The model under review builds one solid part; all positions refer to its coordinate system, in mm. A direction names the side the tool comes from. Coordinates: 2 decimals unless noted, no trailing zeros. Loops run counter-clockwise (first coordinate to the right, second up) from the corner with the lowest first, then second, coordinate; pieces in that order, holes last. Notation, with made-up numbers: M -8,-3 L 32,-3 A31 ccw 32,24 Z; hole C -34,6.5 d8. An arc over 180 degrees is marked long. Use one line per item in the form item = value.
```python
from build123d import *

# Parameters (mm, degrees)
SKETCH_1_W                   = 50
SKETCH_1_H                   = 7
CUT_EXTRUDE_1_DEPTH          = 4
CUT_EXTRUDE_2_DEPTH          = 8
EXTRUDE_1_DEPTH              = 8
EXTRUDE_2_DEPTH              = 8
EXTRUDE_3_DEPTH              = 8
EXTRUDE_4_DEPTH              = 8
EXTRUDE_5_DEPTH              = 8
EXTRUDE_6_DEPTH              = 8
HOLE_WIZARD_M3_1_D           = 3.4
HOLE_WIZARD_M3_1_DEPTH       = 117.890896659
HOLE_WIZARD_M3_1_CBORE_D     = 7
HOLE_WIZARD_M3_1_CBORE_DEPTH = 2.722101968
HOLE_WIZARD_M3_2_D           = 3.4
HOLE_WIZARD_M3_2_DEPTH       = 117.890896659
HOLE_WIZARD_M3_2_CBORE_D     = 7
HOLE_WIZARD_M3_2_CBORE_DEPTH = 2.722101968
HOLE_WIZARD_M3_3_D           = 3.4
HOLE_WIZARD_M3_3_DEPTH       = 99.58962647
HOLE_WIZARD_M3_3_CBORE_D     = 7
HOLE_WIZARD_M3_3_CBORE_DEPTH = 2.722101968
HOLE_WIZARD_3_6_3_6_1_D      = 3.6
HOLE_WIZARD_3_6_3_6_1_DEPTH  = 15
HOLE_WIZARD_3_6_3_6_2_D      = 3.6
HOLE_WIZARD_3_6_3_6_2_DEPTH  = 3
FILLET_1_R                   = 10


with BuildPart() as part:
    # 草图1 → 旋转1 (revolve)
    with BuildSketch(Plane.XZ.offset(-150)):
        with Locations((625, 3.5)):
            Rectangle(SKETCH_1_W, SKETCH_1_H)
    revolve(axis=Axis((600, 150, 7), (0, 0, -1)))

    # 草图2 → 切除-拉伸1 (cut)
    with BuildSketch(Plane.XY.offset(7)):
        with BuildLine():
            ThreePointArc((595.803701911, 199.823599653), (596.702458922, 199.406826168), (596.801488345, 198.421099291))
            ThreePointArc((596.801488345, 198.421099291), (600, 193.5), (603.198511655, 198.421099291))
            ThreePointArc((603.198511655, 198.421099291), (603.297541078, 199.406826168), (604.196298089, 199.823599653))
            ThreePointArc((604.196298089, 199.823599653), (600, 200), (595.803701911, 199.823599653))
        make_face()
    extrude(amount=-CUT_EXTRUDE_1_DEPTH, mode=Mode.SUBTRACT)

    # 草图3 → 切除-拉伸2 (cut, through all)
    with BuildSketch(Plane(origin=(0, 0, 0), x_dir=(-1, 0, 0), z_dir=(0, 0, -1))):
        with BuildLine():
            Line((-613.918146142, 188.239792245), (-619.734819826, 189.794276566))
            ThreePointArc((-619.734819826, 189.794276566), (-638.467982411, 172.2095), (-644.330264345, 147.193717025))
            Line((-644.330264345, 147.193717025), (-640.075704591, 142.93357201))
            ThreePointArc((-640.075704591, 142.93357201), (-639.132532117, 142.101136168), (-638.092310865, 141.393701722))
            Line((-638.092310865, 141.393701722), (-636.23143008, 138.542099914))
            ThreePointArc((-636.23143008, 138.542099914), (-632.908965344, 131), (-628.038547588, 124.351611178))
            Line((-628.038547588, 124.351611178), (-626.499428374, 121.314240241))
            ThreePointArc((-626.499428374, 121.314240241), (-626.406882798, 120.059664989), (-626.157558449, 118.826635745))
            Line((-626.157558449, 118.826635745), (-624.595444519, 113.012006408))
            ThreePointArc((-624.595444519, 113.012006408), (-600, 105.581), (-575.404555481, 113.012006408))
            Line((-575.404555481, 113.012006408), (-573.842441551, 118.826635745))
            ThreePointArc((-573.842441551, 118.826635745), (-573.593117202, 120.059664989), (-573.500571626, 121.314240241))
            Line((-573.500571626, 121.314240241), (-571.961452412, 124.351611178))
            ThreePointArc((-571.961452412, 124.351611178), (-567.091034656, 131), (-563.76856992, 138.542099914))
            Line((-563.76856992, 138.542099914), (-561.907689135, 141.393701722))
            ThreePointArc((-561.907689135, 141.393701722), (-560.867467883, 142.101136168), (-559.924295409, 142.93357201))
            Line((-559.924295409, 142.93357201), (-555.669735655, 147.193717025))
            ThreePointArc((-555.669735655, 147.193717025), (-561.532017589, 172.2095), (-580.265180174, 189.794276566))
            Line((-580.265180174, 189.794276566), (-586.081853858, 188.239792245))
            ThreePointArc((-586.081853858, 188.239792245), (-587.274350681, 187.839198844), (-588.407117509, 187.292058037))
            Line((-588.407117509, 187.292058037), (-591.807117509, 187.106288907))
            ThreePointArc((-591.807117509, 187.106288907), (-600, 188), (-608.192882491, 187.106288907))
            Line((-608.192882491, 187.106288907), (-611.592882491, 187.292058037))
            ThreePointArc((-611.592882491, 187.292058037), (-612.725649319, 187.839198844), (-613.918146142, 188.239792245))
        make_face()
    extrude(amount=-CUT_EXTRUDE_2_DEPTH, mode=Mode.SUBTRACT)

    # 草图4 → 凸台-拉伸1 (add)
    with BuildSketch(Plane.XY.offset(7)):
        with BuildLine():
            Line((595.862693304, 199.826816745), (595.862693304, 194.867524502))
            Line((595.862693304, 194.867524502), (583.669556596, 194.867524502))
            Line((583.669556596, 194.867524502), (582.898992834, 196.984631039))
            ThreePointArc((582.898992834, 196.984631039), (589.257154079, 198.832276841), (595.803701911, 199.823599653))
            ThreePointArc((595.803701911, 199.823599653), (595.833173844, 199.825643938), (595.862693304, 199.826816745))
        make_face()
    extrude(amount=EXTRUDE_1_DEPTH)

    # 草图5 → 凸台-拉伸2 (add)
    with BuildSketch(Plane.XY.offset(7)):
        with BuildLine():
            Line((617.101007166, 196.984631039), (616.330443404, 194.867524502))
            Line((616.330443404, 194.867524502), (604.137306696, 194.867524502))
            Line((604.137306696, 194.867524502), (604.137306696, 199.826816745))
            ThreePointArc((604.137306696, 199.826816745), (604.166826156, 199.825643938), (604.196298089, 199.823599653))
            ThreePointArc((604.196298089, 199.823599653), (610.742845921, 198.832276841), (617.101007166, 196.984631039))
        make_face()
    extrude(amount=EXTRUDE_2_DEPTH)

    # 草图6 → 凸台-拉伸3 (add)
    with BuildSketch(Plane.XY.offset(7)):
        with BuildLine():
            Line((563.212237324, 123.983225047), (569.308805678, 113.423658906))
            Line((569.308805678, 113.423658906), (567.860619516, 111.697777844))
            ThreePointArc((567.860619516, 111.697777844), (563.061475995, 116.302144811), (558.915878003, 121.502720836))
            Line((558.915878003, 121.502720836), (563.212237324, 123.983225047))
        make_face()
    extrude(amount=EXTRUDE_3_DEPTH)

    # 草图7 → 凸台-拉伸4 (add)
    with BuildSketch(Plane.XY.offset(7)):
        with BuildLine():
            Line((559.074930628, 131.149250451), (554.778571307, 128.66874624))
            ThreePointArc((554.778571307, 128.66874624), (552.347539351, 134.859227428), (550.759612349, 141.317591117))
            Line((550.759612349, 141.317591117), (552.978362274, 141.708816592))
            Line((552.978362274, 141.708816592), (559.074930628, 131.149250451))
        make_face()
    extrude(amount=EXTRUDE_4_DEPTH)

    # 草图8 → 凸台-拉伸5 (add)
    with BuildSketch(Plane.XY.offset(7)):
        with BuildLine():
            Line((640.925069372, 131.149250451), (647.021637726, 141.708816592))
            Line((647.021637726, 141.708816592), (649.240387651, 141.317591117))
            ThreePointArc((649.240387651, 141.317591117), (647.652460649, 134.859227428), (645.221428693, 128.66874624))
            Line((645.221428693, 128.66874624), (640.925069372, 131.149250451))
        make_face()
    extrude(amount=EXTRUDE_5_DEPTH)

    # 草图9 → 凸台-拉伸6 (add)
    with BuildSketch(Plane.XY.offset(7)):
        with BuildLine():
            Line((636.787762676, 123.983225047), (641.084121997, 121.502720836))
            ThreePointArc((641.084121997, 121.502720836), (636.938524005, 116.302144811), (632.139380484, 111.697777844))
            Line((632.139380484, 111.697777844), (630.691194322, 113.423658906))
            Line((630.691194322, 113.423658906), (636.787762676, 123.983225047))
        make_face()
    extrude(amount=EXTRUDE_6_DEPTH)

    # M3 六角头机械螺钉的柱形沉头孔1
    with Locations(Plane(origin=(427.993971004, -247.10243437, 0), x_dir=(0, 0, -1), z_dir=(0.866025404, -0.5, 0))):
        with Locations((-11, 420.010928076), (-11, 439.796693059)):
            CounterBoreHole(HOLE_WIZARD_M3_1_D / 2, HOLE_WIZARD_M3_1_CBORE_D / 2, HOLE_WIZARD_M3_1_CBORE_DEPTH, depth=HOLE_WIZARD_M3_1_DEPTH)

    # M3 六角头机械螺钉的柱形沉头孔2
    with Locations(Plane(origin=(472.006028996, 272.5128079, 0), x_dir=(0, 0, 1), z_dir=(-0.866025404, -0.5, 0))):
        with Locations((11, -160.203306941), (11, -179.989071924)):
            CounterBoreHole(HOLE_WIZARD_M3_2_D / 2, HOLE_WIZARD_M3_2_CBORE_D / 2, HOLE_WIZARD_M3_2_CBORE_DEPTH, depth=HOLE_WIZARD_M3_2_DEPTH)

    # M3 六角头机械螺钉的柱形沉头孔3
    with Locations(Plane(origin=(0, 199.58962647, 0), x_dir=(1, 0, 0), z_dir=(0, 1, 0))):
        with Locations((609.892882491, -11), (590.107117509, -11)):
            CounterBoreHole(HOLE_WIZARD_M3_3_D / 2, HOLE_WIZARD_M3_3_CBORE_D / 2, HOLE_WIZARD_M3_3_CBORE_DEPTH, depth=HOLE_WIZARD_M3_3_DEPTH)

    # Ø3.6 (3.6) 直径孔1
    with Locations(Plane(origin=(0, 0, 0), x_dir=(-1, 0, 0), z_dir=(0, 0, -1))):
        with Locations((-600, 103), (-647, 150), (-553, 150)):
            Hole(HOLE_WIZARD_3_6_3_6_1_D / 2, depth=HOLE_WIZARD_3_6_3_6_1_DEPTH)

    # Ø3.6 (3.6) 直径孔2
    with Locations(Plane.XY.offset(3)):
        with Locations((600, 197)):
            Hole(HOLE_WIZARD_3_6_3_6_2_D / 2, depth=HOLE_WIZARD_3_6_3_6_2_DEPTH)

    # 圆角1
    fillet_1_edges = [part.edges().sort_by_distance(p)[0] for p in [
        (580.265180174, 189.794276566, 3.5),
        (555.669735655, 147.193717025, 3.5),
        (575.404555481, 113.012006408, 3.5),
        (624.595444519, 113.012006408, 3.5),
        (644.330264345, 147.193717025, 3.5),
        (619.734819826, 189.794276566, 3.5),
    ]]
    fillet(fillet_1_edges, radius=FILLET_1_R)


solid = part.part
```
1. Insertion check: P1, Ø8, axis at x = 565.5, z = 10, coming from the +Y side; P2, Ø6.5, axis at x = 609.5, z = 10.5, coming from the -Y side; P3, Ø3, axis at y = 133, z = 4.5, coming from the +X side. Each pin has a flat end and moves straight along its axis. Give the tip position at first contact, or say it passes through.
Response values:
P1 = 188.54
P2 = 194.87
P3 = 647.54
2. Add section A-A (x = 600). State the section outline as (y, z) points, then the cut area to 3 significant figures.
Response values:
outline = M 100,0 L 101.2,0 L 101.2,7 L 100,7 Z; M 104.8,0 L 105.58,0 L 105.58,7 L 104.8,7 Z; M 188,0 L 195.2,0 L 195.2,3 L 193.5,3 L 193.5,7 L 188,7 Z; M 198.8,0 L 200,0 L 200,3 L 198.8,3 Z
area = 61.1 mm^2
3. Machinability: for faces 1 (the face through (589, 196.868, 13)), 2 (the face through (599.9, 193.5, 5)), 3 (the face through (626.41, 120.08, 3.45)), 4 (the face through (643.83, 134.2, 10.63)), 5 (the face through (566.895, 117.604, 10.055)), which of the approach directions +Z, -Z, +X, -X, +Y, -Y give a long, thin tool a straight path to every point of the face, cutting with its end or side? Answer none if there is none.
Response values:
face_1 = +Y
face_2 = +Z
face_3 = +Z, -Z
face_4 = none
face_5 = +Z, +Y
4. Add section C-C (y = 172.5). State the section outline as (x, z) points, then the cut area to 3 significant figures.
Response values:
outline = M 555.35,0 L 561.7,0 L 561.7,7 L 555.35,7 Z; M 638.3,0 L 644.65,0 L 644.65,7 L 638.3,7 Z
area = 88.9 mm^2
5. Wall thickness on line 1 along Y through (x, z) = (600, 5.75); line 2 along X through (y, z) = (150, 4.25); line 3 along Z through (x, y) = (555, 141.5): over which ranges is each line inside the solid? List them lowest first. Write a range as from..to.
Response values:
line_1 = 100..101.2, 104.8..105.58, 188..193.5
line_2 = 550..551.2, 554.8..555.71, 644.29..645.2, 648.8..650
line_3 = 0..7
6. The part is to be moulded in two halves that separate along Z. For faces 6 (the face through (609, 197, 15)), 7 (the face through (638.3, 172.5, 3.5)), 8 (the face through (644.76, 131.636, 11.759)), say which applies: pulls with the +Z half, pulls with the -Z half, needs draft (parallel to the pull), parting line crosses it, or undercut.
Response values:
face_6 = pulls with the +Z half
face_7 = needs draft
face_8 = undercut
7. Add section D-D (y = 103). State the section outline as (x, z) points, then the cut area to 3 significant figures.
Response values:
outline = M 582.94,0 L 598.2,0 L 598.2,7 L 582.94,7 Z; M 601.8,0 L 617.06,0 L 617.06,7 L 601.8,7 Z
area = 214 mm^2
8. Add section B-B (y = 150). State the section outline as (x, z) points, then the cut area to 3 significant figures.
Response values:
outline = M 550,0 L 551.2,0 L 551.2,7 L 550,7 Z; M 554.8,0 L 555.71,0 L 555.71,7 L 554.8,7 Z; M 644.29,0 L 645.2,0 L 645.2,7 L 644.29,7 Z; M 648.8,0 L 650,0 L 650,7 L 648.8,7 Z
area = 29.5 mm^2
